Build history of the part. All positions in model axes, mm. Face numbers are marked on the shaded views. A direction names the side the tool comes from. Round coordinates to 2 decimals unless told otherwise and drop trailing zeros. Write each loop counter-clockwise with the first axis right and the second up, starting at its lowest first coordinate (ties: lowest second). Pieces come first, ordered by that corner, then holes. Notation, with made-up numbers: M 63,35 L 93,35 A34 ccw 93,67 Z; hole C 23,26.5 d10. An arc over 180 degrees is marked long. Write item = value, one per line.
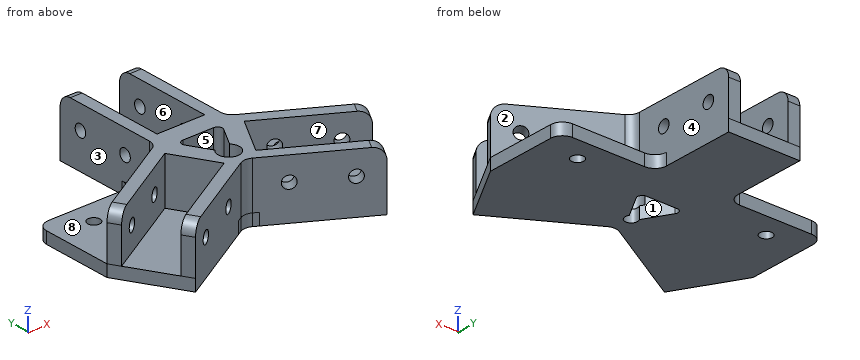
from build123d import *

# Parameters (mm, degrees)
F1_DEPTH    = 20
F2_R        = 2.6
F3_DEPTH    = 50.6016350946
F4_COUNT    = 3
F4_ANGLE    = 240
F6_DEPTH    = 5
F7_T1_DEPTH = 25
F10_DEPTH   = 5
F11_DEPTH   = 25.001
F12_R       = 2
F13_R       = 2.6
F14_DEPTH   = 25.001
F15_R       = 5
F16_R       = 4.5
F17_DEPTH   = 20


# Not quite as in the source:
# - a fillet or chamfer that OpenCascade refuses, or shapes differently, is made with other operations: its cross-section is extruded or revolved along the edge and cut away or added


with BuildPart() as f1:
    # F0 (on Top) → F1 (new body)
    with BuildSketch(Plane.XY):
        Polygon((43.0992290895, -36.5458269543), (6.7261621305, -15.5458269543), (16.8261621305, 1.9478862021), (53.1992290895, -19.0521137979), (55.6992290895, -14.7219867789), (14.8979589003, 8.8346375481), (0, 0), (-0.2020410997, -17.3193296462), (40.5992290895, -40.8759539732), align=None)
    extrude(amount=F1_DEPTH)

    # F2 (on face) → F3 (cut, through all)
    with BuildSketch(Plane(origin=(-7.55, -13.0769835971, 0), x_dir=(0.8660254038, -0.5, 0), z_dir=(-0.5, -0.8660254038, 0))):
        with Locations((45.5979407522, 10)):
            Circle(F2_R)
        with Locations((23.5979407522, 10)):
            Circle(F2_R)
    extrude(amount=-F3_DEPTH, mode=Mode.SUBTRACT)

    # F4: F1 ×3 about axis
    f4_axis = Axis((0, 0, 10), (0, 0, -1))


with BuildPart() as f1_1:
    add(f1.part)
    for i in range(1, F4_COUNT):
        add(f1.part.rotate(f4_axis, i * F4_ANGLE / (F4_COUNT - 1)))

    # F5 (on face) → F6 (join)
    with BuildSketch(Plane(origin=(0, 0, 0), x_dir=(1, 0, 0), z_dir=(0, 0, -1))):
        Polygon((0, 17.4359781295), (-40.5992290895, 40.8759539732), (-55.6992290895, 14.7219867789), (-15.1, -8.7179890648), (-15.1, -55.5979407522), (15.1, -55.5979407522), (15.1, -8.7179890648), (55.6992290895, 14.7219867789), (40.5992290895, 40.8759539732), align=None)
    extrude(amount=F6_DEPTH)

    # F7: fillet of radius 5 on 3 edges, made by hand

    # F7_s2 → F7_t1 (join)
    with BuildSketch(Plane.XY.offset(-5)):
        with BuildLine():
            ThreePointArc((2.5, -18.8792383324), (0, -18.2093653514), (-2.5, -18.8792383324))
            Line((-2.5, -18.8792383324), (-2.55, -18.7926357921))
            ThreePointArc((-2.55, -18.7926357921), (-1.299975, -18.0710489919), (-0.05, -17.3493755891))
            Line((-0.05, -17.3493755891), (0.05, -17.3493755891))
            ThreePointArc((0.05, -17.3493755891), (1.299975, -18.0710489919), (2.55, -18.7926357921))
            Line((2.55, -18.7926357921), (2.5, -18.8792383324))
        make_face()
        with BuildLine():
            ThreePointArc((15.0999, 11.6046826757), (15.7697729811, 9.1046826757), (17.5999, 7.2745556568))
            Line((17.5999, 7.2745556568), (17.5499, 7.1879531164))
            ThreePointArc((17.5499, 7.1879531164), (16.299975, 7.9097131217), (15.05, 8.6313865244))
            Line((15.05, 8.6313865244), (15, 8.7179890648))
            ThreePointArc((15, 8.7179890648), (15, 10.1613358702), (14.9999, 11.6046826757))
            Line((14.9999, 11.6046826757), (15.0999, 11.6046826757))
        make_face()
        with BuildLine():
            ThreePointArc((-17.5999, 7.2745556568), (-15.7697729811, 9.1046826757), (-15.0999, 11.6046826757))
            Line((-15.0999, 11.6046826757), (-14.9999, 11.6046826757))
            ThreePointArc((-14.9999, 11.6046826757), (-15, 10.1613358702), (-15, 8.7179890648))
            Line((-15, 8.7179890648), (-15.05, 8.6313865244))
            ThreePointArc((-15.05, 8.6313865244), (-16.299975, 7.9097131217), (-17.5499, 7.1879531164))
            Line((-17.5499, 7.1879531164), (-17.5999, 7.2745556568))
        make_face()
    extrude(amount=F7_T1_DEPTH)

    # F9 (on face) → F10 (join)
    with BuildSketch(Plane(origin=(0, 0, -5), x_dir=(1, 0, 0), z_dir=(0, 0, -1))):
        with BuildLine():
            Line((-55.6992290895, 14.7219867789), (-55.6992290895, -20))
            Line((-55.6992290895, -20), (55.6992290895, -20))
            Line((55.6992290895, -20), (55.6992290895, 14.7219867789))
            Line((55.6992290895, 14.7219867789), (52.6519667355, 20))
            Line((52.6519667355, 20), (4.4410161514, 20))
            Line((4.4410161514, 20), (2.5, 18.8793538025))
            ThreePointArc((2.5, 18.8793538025), (0, 18.2094808214), (-2.5, 18.8793538025))
            Line((-2.5, 18.8793538025), (-4.4410161514, 20))
            Line((-4.4410161514, 20), (-52.6519667355, 20))
            Line((-52.6519667355, 20), (-55.6992290895, 14.7219867789))
        make_face()
    extrude(amount=-F10_DEPTH)

    # F8 (on face) → F11 (cut, through all)
    with BuildSketch(Plane.XY.offset(20)):
        Polygon((10, 5.0614941438), (-10, 5.0614941438), (0, -12.2590139319), align=None)
    extrude(amount=-F11_DEPTH, mode=Mode.SUBTRACT)

    # F12
    f12_edges = [f1_1.edges().sort_by_distance(p)[0] for p in [
        (10, 5.061494, 7.5),
        (-10, 5.061494, 7.5),
        (0, -12.259014, 7.5),
    ]]
    fillet(f12_edges, radius=F12_R)

    # F13 (on face) → F14 (cut, through all)
    with BuildSketch(Plane(origin=(0, 0, -5), x_dir=(1, 0, 0), z_dir=(0, 0, -1))):
        with Locations((-40, -10)):
            Circle(F13_R)
        with Locations((40, -10)):
            Circle(F13_R)
        with Locations((0, 10)):
            Circle(F13_R)
    extrude(amount=-F14_DEPTH, mode=Mode.SUBTRACT)

    # F15
    f15_edges = [f1_1.edges().sort_by_distance(p)[0] for p in [
        (-15.1, 20, -2.5),
        (15.1, 20, -2.5),
        (55.699229, 20, -2.5),
        (-55.699229, 20, -2.5),
        (-12.6, 55.597941, 20),
        (12.6, 55.597941, 20),
        (-54.449229, -16.88705, 20),
        (-41.849229, -38.71089, 20),
        (54.449229, -16.88705, 20),
        (41.849229, -38.71089, 20),
    ]]
    fillet(f15_edges, radius=F15_R)

    # F16 (on face) → F17 (cut)
    with BuildSketch(Plane.XY.offset(20)):
        with Locations((0, -10)):
            Circle(F16_R)
    extrude(amount=-F17_DEPTH, mode=Mode.SUBTRACT)


solid = f1_1.part
1. Mould opens along X. For the marked faces 1, 2 and 3 say: pulls with the +X half, pulls with the -X half, needs draft (parallel to the pull), parting line crosses it, or undercut.
Responses:
face_1 = undercut
face_2 = pulls with the +X half
face_3 = pulls with the -X half
2. Band-saw the part on A-A (y = 10). List the corners of the cut face in (x, z).
Responses:
outline = M -55.7,-5 L -42.6,-5 L -42.6,0 L -55.7,0 Z; M -37.4,-5 L 37.4,-5 L 37.4,0 L 15.36,0 L 15.36,20 L -15.36,20 L -15.36,0 L -37.4,0 Z; M 42.6,-5 L 55.7,-5 L 55.7,0 L 42.6,0 Z
3. Probe probe 1 along X at (y, z) = (10, -1.25); probe 2 along Y at (x, z) = (13, 8); probe 3 along X at (y, z) = (18.5, 9.25). List the from-to ranges inside material, lowest first.
Responses:
probe_1 = -55.7 to -42.6, -37.4 to 37.4, 42.6 to 55.7
probe_2 = -21.36 to -19.17, -4.68 to 21.94, 25.26 to 43.94, 47.26 to 55.6
probe_3 = -15.1 to -10.1, 10.1 to 15.1
4. Flat gauge pins, fed straight in: pin 1 (1.5 mm diameter, centred on y = 45.5, z = 11, fed in from +X); pin 2 (1.5 mm diameter, centred on x = 41.5, z = -2, fed in from +Y); pin 3 (8 mm diameter, centred on y = -26.5, z = 4.5, fed in from +X); pin 4 (12 mm diameter, centred on y = 26, z = 9, fed in from +X). Where does each tip first touch, or does it go through?
Responses:
pin_1 = through
pin_2 = 20
pin_3 = 32.63
pin_4 = 15.1
5. Tool access for the marked faces 4, 5, 6, 7 and 8: list every direction of +Z, -Z, +X, -X, +Y, -Y with a clear straight run to the whole face (end or side of a thin tool).
Responses:
face_4 = +Z, +X, +Y
face_5 = +Z, -Z
face_6 = +Z, +Y
face_7 = +Z
face_8 = +Z, -X, +Y
